Check sheet for the drawn part. Datum: minimum x, y, z corner. Units: mm. Round coordinates to 2 decimals unless told otherwise and drop trailing zeros. Write each loop counter-clockwise with the first axis right and the second up, starting at its lowest first coordinate (ties: lowest second). Pieces come first, ordered by that corner, then holes. Notation, with made-up numbers: (18, 80.25) - (34, 80.25) arc R17 ccw to (34, 101.25) - close; hole circle Ø3 at (2.5, 36). An arc over 180 degrees is marked (long way). Answer as a JSON object with one key per item and string values.
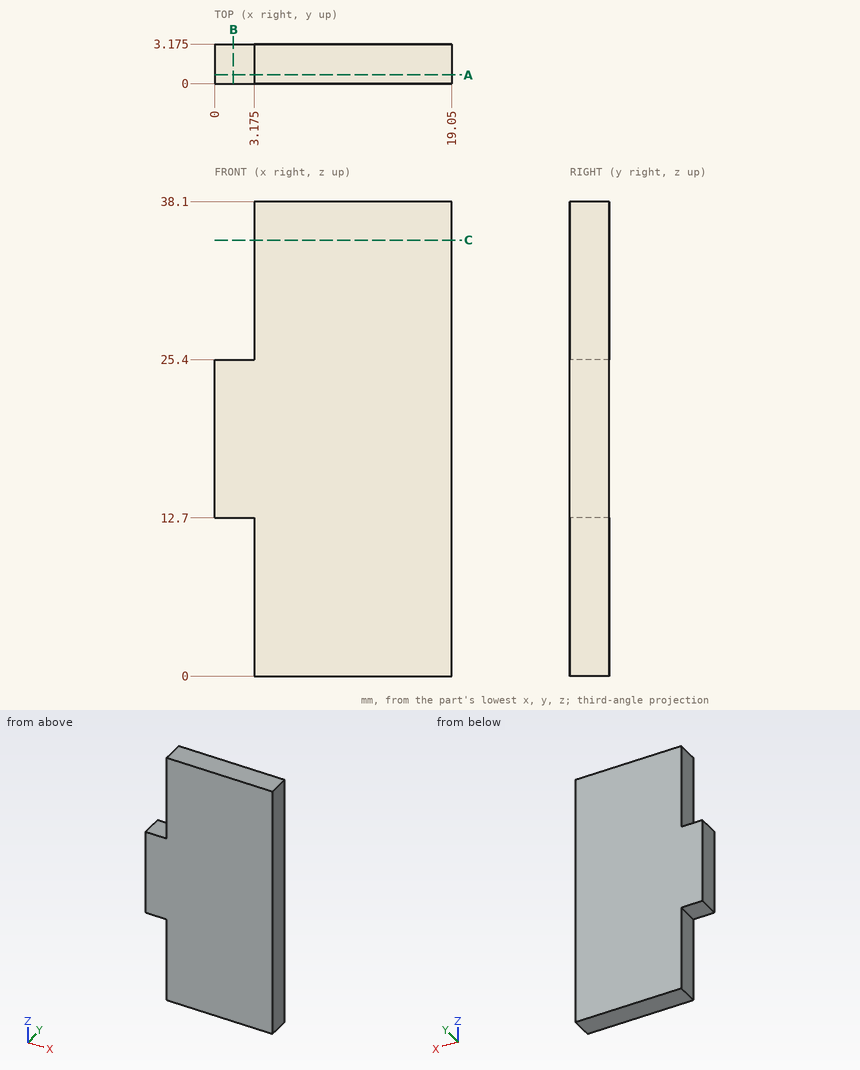
1. Cross-section at B-B (x = 1.5). Record the boundary of the cut face in (y, z) (3 decimals), plus the area to 3 significant figures.
Completed:
{"outline": "(0, 12.7) - (3.175, 12.7) - (3.175, 25.4) - (0, 25.4) - close", "area": "40.3 mm^2"}
2. Go/stop test with a flat-tipped pin: pin 1 (1.6 mm diameter, centred on x = 2, y = 2, fed in from +Z). Record where the tip stops, or that it passes through.
Completed:
{"pin 1": "stops at z = 25.4"}
3. Cross-section at C-C (z = 35). Record the boundary of the cut face in (x, y) (3 decimals), plus the area to 3 significant figures.
Completed:
{"outline": "(3.175, 0) - (19.05, 0) - (19.05, 3.175) - (3.175, 3.175) - close", "area": "50.4 mm^2"}
4. Material ranges on probe 1 along X at (y, z) = (0.9, 30.5) (3 decimals); probe 2 along Z at (x, y) = (1.75, 1.2), recorded low to high. Write a range as from..to.
Completed:
{"probe 1": "x = 3.175..19.05", "probe 2": "z = 12.7..25.4"}
5. Cross-section at A-A (y = 0.7). Record the boundary of the cut face in (x, z) (3 decimals), plus the area to 3 significant figures.
Completed:
{"outline": "(0, 12.7) - (3.175, 12.7) - (3.175, 0) - (19.05, 0) - (19.05, 38.1) - (3.175, 38.1) - (3.175, 25.4) - (0, 25.4) - close", "area": "645 mm^2"}
